```python
from build123d import *

# Parameters (mm, degrees)
F4_W          = 300
F4_H          = 8
F0_DEPTH      = 75
F5_DEPTH      = 25
F6_D          = 8
F7_W          = 85
F7_H          = 23.832924
F3_DEPTH      = 10
F3_DEPTH_BACK = 18


with BuildPart() as f0:
    # F4 (on Front) → F0 (new body)
    with BuildSketch(Plane.XZ):
        with Locations((-150, -4)):
            Rectangle(F4_W, F4_H)
    extrude(amount=F0_DEPTH)

    # F1 (on face) → F5 (cut)
    with BuildSketch(Plane.XY):
        with BuildLine():
            Line((0, 0), (-300, 0))
            ThreePointArc((-300, 0), (-150, -31.167076), (0, 0))
        make_face()
    extrude(amount=-F5_DEPTH, mode=Mode.SUBTRACT)

    # F6 (through all)
    with Locations(Plane.XY):
        with Locations((-270, -53), (-250, -53), (-230.000013, -53), (-210.000013, -53), (-90, -53), (-70, -53), (-50, -53), (-30, -53)):
            Hole(F6_D / 2)

    # F7 (on face) → F3 (join, two sides)
    with BuildSketch(Plane.XY) as f3_sk:
        with Locations((-150, -53.083538)):
            Rectangle(F7_W, F7_H)
    extrude(amount=F3_DEPTH)
    extrude(f3_sk.sketch, amount=-F3_DEPTH_BACK)


solid = f0.part
```
Geometry check sheet. Reference: the model listing, model coordinates, mm. A direction names the side the tool comes from. Coordinates: 2 decimals unless noted, no trailing zeros. Order: outer loops, then holes, each group sorted by start corner. A loop starts at its lowest first (then second) coordinate and runs counter-clockwise, first axis right, second up. Notation, with made-up numbers: M 12.5,53.25 L 65.5,53.25 A21 ccw 65.5,75.25 Z; hole C 58,-3.75 d9. An arc over 180 degrees is marked long. Answer as a JSON object with one key per item and string values.
Q1. Scan lines: line 1 (Z direction, x = -232.5, y = -25); line 2 (Y direction, x = -247, z = -2); line 3 (Y direction, x = -50, z = -2.5). Record each from-to range of solid material in increasing order.
Results are:
{"line 1": "z = -8 to 0", "line 2": "y = -75 to -55.65, -50.35 to -18.46", "line 3": "y = -75 to -57, -49 to -17.65"}
Q2. Release check for a two-part mould opening along X. For faces 1 (the cylindrical face through (-152.16, -31.16, -3.94)), 2 (the flat face through (-107.5, -53, 5)), 3 (the flat face through (-152, -75, -4)) record: released by +X, released by -X, zero draft, split by the parting line, or undercut.
Results are:
{"face 1": "undercut", "face 2": "released by +X", "face 3": "zero draft"}
Q3. Cross-section at B-B on y = -28. Record the cut outline in (x, z).
Results are:
{"outline": "M -300,-8 L -198.73,-8 L -198.73,0 L -300,0 Z; M -101.27,-8 L 0,-8 L 0,0 L -101.27,0 Z"}
Q4. Cross-section at C-C on x = -250. Record the cut outline in (y, z).
Results are:
{"outline": "M -75,-8 L -57,-8 L -57,0 L -75,0 Z; M -49,-8 L -17.65,-8 L -17.65,0 L -49,0 Z"}
Q5. Tool access check on faces 4 (the flat face through (-151, -65, -13)), 5 (the flat face through (-151, -65, 5)), 6 (the flat face through (-151, -41.167, -13)). Record the directions out of +Z, -Z, +X, -X, +Y, -Y that give a thin tool (end or side, any length) a straight path to the whole face; none if there is none.
Results are:
{"face 4": "-Z, +X, -X, -Y", "face 5": "+Z, +X, -X, -Y", "face 6": "-Z, +X, -X, +Y"}
Q6. Depth check by flat-ended pin: pin 1 Ø5 at (y, z) = (-55.5, -12.5) entering from -X; pin 2 Ø9 at (x, y) = (-90, -53) entering from +Z; pin 3 Ø5 at (x, z) = (-130.5, -12.5) entering from -Y. Enter the tip coordinate at first touch or a pass-through.
Results are:
{"pin 1": "stops at x = -192.5", "pin 2": "stops at z = 0", "pin 3": "stops at y = -65"}
Q7. Cross-section at A-A on z = -5.25. Give the number of separate pieces and of enclosed holes in the cut face, and give its area (3 significant figures).
Results are:
{"separate pieces": "1", "enclosed holes": "8", "area": "15,800 mm²"}
